Source: three-view drawing plus pictorial views. Frame: mm from the lowest corner of the part. A direction names the side the tool comes from. Give positions to 0.01 mm unless a question says otherwise; leave off trailing zeros. Loops run counter-clockwise (first coordinate to the right, second up) from the corner with the lowest first, then second, coordinate; pieces in that order, holes last.
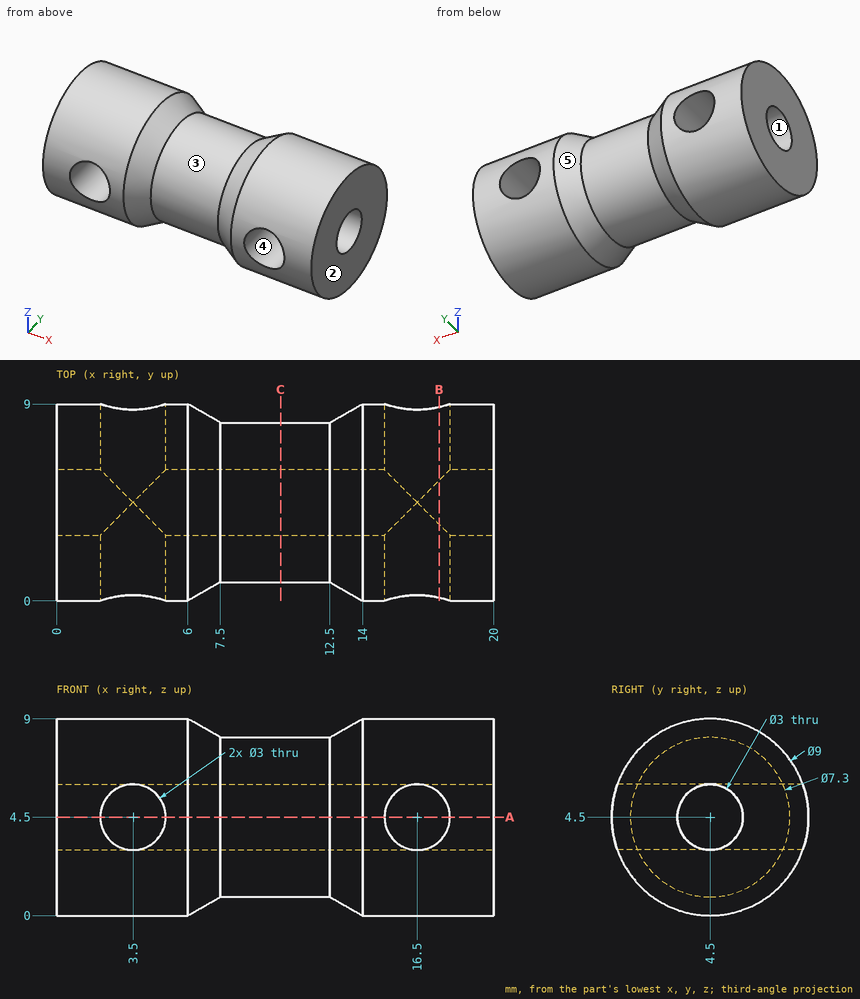
(1) Reachability of the marked faces 4 and 5 from +Z, -Z, +X, -X, +Y, -Y: full face, straight path, thin tool, end or side. Return the list, or none.
Values follow:
face 4: +Y, -Y
face 5: none
(2) Cut plane B-B (x = 17.5). Return the cut outline in (y, z), and give its area (3 significant figures).
Values follow:
outline: (0.14, 3.38) arc R4.5 ccw to (8.86, 3.38) - (5.5, 3.38) arc R1.5 cw to (3.5, 3.38) - close; (0.14, 5.62) - (3.5, 5.62) arc R1.5 cw to (5.5, 5.62) - (8.86, 5.62) arc R4.5 ccw to start
area: 42.7 mm2
(3) Cut plane A-A (z = 4.5). Count the separate pieces of the cut face and the enclosed holes in it, and give its area (4 significant figures).
Values follow:
separate pieces: 6
enclosed holes: 0
area: 72.95 mm2
(4) Cut plane C-C (x = 10.25). Return the cut outline in (y, z).
Values follow:
outline: circle Ø7.3 at (4.5, 4.5); hole circle Ø3 at (4.5, 4.5)
(5) Mould query, pull axis Z, two halves, no side actions, for the marked faces 1, 2 and 3. Classes: +Z half, -Z half, draft (parallel to the pull), parting line (faces both ways), or undercut.
Values follow:
face 1: undercut
face 2: draft
face 3: parting line
(6) Ray query, probe 1 along X at (y, z) = (0.75, 3.5); probe 2 along X at (y, z) = (8, 5.75); probe 3 along Z at (x, y) = (3.5, 2.45). Return the intervals inside material, ascending.
Values follow:
probe 1: x = 0 to 2.38, 4.62 to 7.09, 12.91 to 15.38, 17.62 to 20
probe 2: x = 0 to 2.67, 4.33 to 7.38, 12.62 to 15.67, 17.33 to 20
probe 3: z = 0.49 to 3, 6 to 8.51
